```python
from build123d import *

# Parameters (mm, degrees)
F1_DEPTH = 13
F4_DEPTH = 34.5
F5_DEPTH = 13
F6_DEPTH = 15.6
F7_DEPTH = 5.01


with BuildPart() as f1:
    # F0 (on Right) → F1 (new body)
    with BuildSketch(Plane.YZ):
        Polygon((-37.0099544525, -6.5021011516), (-28.6699544525, -6.5021011516), (-28.6699544525, -4.9721011516), (-31.7186098982, -1.9396598952), (-28.6861686418, 1.1089955505), (-20.5187435475, 1.1084489664), (-20.4991411365, 6.4742991461), (-34.9424730613, 6.4934650898), (-37.0099544525, 1.4721968726), (-37.0099544525, -2.5149521395), align=None)
        Polygon((-37.0099544525, 6.4934650898), (-37.0099544525, 1.4721968726), (-34.9424730613, 6.4934650898), align=None)
    extrude(amount=F1_DEPTH)

    # F3: F1 across face


with BuildPart() as f1_1:
    add(f1.part)
    add(f1.part.mirror(Plane(origin=(6.5, -20.508942342, 3.7913740563), x_dir=(-1, 0, 0), z_dir=(0, 0.9999933272, -0.0036531546))))

    # F2 (on face) → F4 (cut)
    with BuildSketch(Plane.XZ.offset(37.0099544525)):
        with BuildLine():
            ThreePointArc((9.075, 0), (8.3207999616, 1.8207999616), (6.5, 2.575))
            Line((6.5, 2.575), (6.5, 0))
            Line((6.5, 0), (9.075, 0))
        make_face()
        with BuildLine():
            ThreePointArc((6.5, 2.575), (4.6792000384, 1.8207999616), (3.925, 0))
            Line((3.925, 0), (6.5, 0))
            Line((6.5, 0), (6.5, 2.575))
        make_face()
        with BuildLine():
            Line((6.5, 0), (3.925, 0))
            ThreePointArc((3.925, 0), (4.6792000384, -1.8207999616), (6.5, -2.575))
            Line((6.5, -2.575), (6.5, 0))
        make_face()
        with BuildLine():
            Line((6.5, 0), (6.5, -2.575))
            ThreePointArc((6.5, -2.575), (8.3207999616, -1.8207999616), (9.075, 0))
            Line((9.075, 0), (6.5, 0))
        make_face()
    extrude(amount=-F4_DEPTH, mode=Mode.SUBTRACT)

    # F0 (on Right) → F5 (join)
    with BuildSketch(Plane.YZ):
        Polygon((-39.0099544525, 0.4721968726), (-37.0099544525, -2.5149521395), (-37.0099544525, 1.4721968726), (-39.0099544525, 1.4721968726), align=None)
        Polygon((-39.0099544525, 1.4721968726), (-37.0099544525, 1.4721968726), (-37.0099544525, 6.4934650898), align=None)
    extrude(amount=F5_DEPTH)

    # F2 (on face) → F6 (cut)
    with BuildSketch(Plane.XZ.offset(37.0099544525)):
        with BuildLine():
            ThreePointArc((9.075, 0), (8.3207999616, 1.8207999616), (6.5, 2.575))
            Line((6.5, 2.575), (6.5, 0))
            Line((6.5, 0), (9.075, 0))
        make_face()
        with BuildLine():
            ThreePointArc((6.5, 2.575), (4.6792000384, 1.8207999616), (3.925, 0))
            Line((3.925, 0), (6.5, 0))
            Line((6.5, 0), (6.5, 2.575))
        make_face()
        with BuildLine():
            Line((6.5, 0), (3.925, 0))
            ThreePointArc((3.925, 0), (4.6792000384, -1.8207999616), (6.5, -2.575))
            Line((6.5, -2.575), (6.5, 0))
        make_face()
        with BuildLine():
            Line((6.5, 0), (6.5, -2.575))
            ThreePointArc((6.5, -2.575), (8.3207999616, -1.8207999616), (9.075, 0))
            Line((9.075, 0), (6.5, 0))
        make_face()
    extrude(amount=F6_DEPTH, mode=Mode.SUBTRACT)

    # F2 (on face) → F7 (cut)
    with BuildSketch(Plane.XZ.offset(37.0099544525)):
        with BuildLine():
            Line((6.5, 6.4934650898), (3.925, 6.4934650898))
            Line((3.925, 6.4934650898), (3.925, 0))
            ThreePointArc((3.925, 0), (4.6792000384, 1.8207999616), (6.5, 2.575))
            Line((6.5, 2.575), (6.5, 6.4934650898))
        make_face()
        with BuildLine():
            Line((9.075, 6.4934650898), (6.5, 6.4934650898))
            Line((6.5, 6.4934650898), (6.5, 2.575))
            ThreePointArc((6.5, 2.575), (8.3207999616, 1.8207999616), (9.075, 0))
            Line((9.075, 0), (9.075, 6.4934650898))
        make_face()
        with BuildLine():
            ThreePointArc((9.075, 0), (8.3207999616, -1.8207999616), (6.5, -2.575))
            Line((6.5, -2.575), (6.5, -6.5021011516))
            Line((6.5, -6.5021011516), (9.075, -6.5021011516))
            Line((9.075, -6.5021011516), (9.075, 0))
        make_face()
        with BuildLine():
            ThreePointArc((6.5, -2.575), (4.6792000384, -1.8207999616), (3.925, 0))
            Line((3.925, 0), (3.925, -6.5021011516))
            Line((3.925, -6.5021011516), (6.5, -6.5021011516))
            Line((6.5, -6.5021011516), (6.5, -2.575))
        make_face()
    extrude(amount=F7_DEPTH, mode=Mode.SUBTRACT)


solid = f1_1.part
```
CAD build for the part. Positions are in the model's coordinates, mm. A direction names the side the tool comes from. Coordinates: 2 decimals unless noted, no trailing zeros. Order: outer loops, then holes, each group sorted by start corner. A loop starts at its lowest first (then second) coordinate and runs counter-clockwise, first axis right, second up. Notation, with made-up numbers: (13, -19) - (61, -19) arc R18 cw to (61, 11) - close; hole circle Ø3 at (45.25, 16). An arc over 180 degrees is marked (long way). Answer in a Markdown table with one row per item.
1. Drill centre lines: L1, parallel to X at y = -36.5, z = -1.5; L2, parallel to Y at x = 9.5, z = 0.75; L3, parallel to Y at x = 4.5, z = 3. Where is each one in solid material? Low to high. Write a range as from..to.
Answer:
| item | result |
|---|---|
| L1 | 0..4.41, 8.59..13 |
| L2 | -39.01..-29.04, -12.06..-4.03 |
| L3 | -37.01..-4.01 |
2. Flat gauge pins, fed straight in: P1, Ø6.5, axis at x = 5.5, y = -34.5, coming from the -Z side; P2, Ø1, axis at y = -38, z = 3, coming from the -X side; P3, Ø1, axis at x = 6.5, y = -11.5, coming from the -Z side; P4, Ø1, axis at y = -17, z = -1, coming from the -X side. Where does each tip first touch, or does it go through?
Answer:
| item | result |
|---|---|
| P1 | z = -6.5 |
| P2 | x = 0 |
| P3 | z = -6.57 |
| P4 | through |
3. Slice it at B-B, the plane y = -9. List the corners of the cut face in (x, z) (3 decimals).
Answer:
| item | result |
|---|---|
| outline | (0, -6.586) - (13, -6.586) - (13, 6.406) - (0, 6.406) - close; hole circle Ø5.15 at (6.5, 0) |
4. Pull direction Y, two halves, no side cores. Call faces 4 (the face through (1.836, -30.224, -0.437)), 5 (the face through (6.41, -30.17, -3.48)), 6 (the face through (6, -37.01, 4)), 7 (the face through (6, -33, -6.502)): +Y half, -Y half, draft (parallel to the pull), parting line (faces both ways), or undercut.
Answer:
| item | result |
|---|---|
| face 4 | undercut |
| face 5 | undercut |
| face 6 | -Y half |
| face 7 | draft |
5. Slice it at C-C, the plane x = 5.75. List the corners of the cut face in (y, z).
Answer:
| item | result |
|---|---|
| outline | (-37.01, -6.5) - (-28.67, -6.5) - (-28.67, -4.97) - (-31.19, -2.46) - (-37.01, -2.46) - close; (-37.01, 2.46) - (-4.02, 2.46) - (-3.99, 6.37) - (-6.06, 6.39) - (-20.5, 6.47) - (-34.94, 6.49) - (-37.01, 6.49) - close; (-12.42, -6.56) - (-4.08, -6.62) - (-4.05, -2.46) - (-9.79, -2.46) - (-12.41, -5.03) - close |
6. Slice it at D-D, the plane x = 1.5. List the corners of the cut face in (y, z).
Answer:
| item | result |
|---|---|
| outline | (-39.01, 0.47) - (-37.01, -2.51) - (-37.01, -6.5) - (-28.67, -6.5) - (-28.67, -4.97) - (-31.72, -1.94) - (-28.69, 1.11) - (-20.52, 1.11) - (-12.35, 1.05) - (-9.34, -2.02) - (-12.41, -5.03) - (-12.42, -6.56) - (-4.08, -6.62) - (-3.99, 6.37) - (-6.06, 6.39) - (-20.5, 6.47) - (-34.94, 6.49) - (-37.01, 6.49) - (-39.01, 1.47) - close |
7. 3-axis set-ups, long thin cutter, end or side, ignore diameter. For faces 1 (the face through (6, -28.67, -6)), 2 (the face through (11.097, -30.224, -0.437)), 3 (the face through (3.925, -38, 2)): which of +Z, -Z, +X, -X, +Y, -Y reach the whole face in a straight line?
Answer:
| item | result |
|---|---|
| face 1 | -Z, +X, -X |
| face 2 | +X, -X |
| face 3 | +Z, -Z, -Y |
8. Slice it at A-A, the plane z = -1. Give the number of separate pieces and of enclosed holes in the cut face, then the cut area to 3 significant figures.
Answer:
| item | result |
|---|---|
| separate pieces | 4 |
| enclosed holes | 0 |
| area | 111 mm² |
